from build123d import *

# Parameters (mm, degrees)
SKETCH1_R           = 12.5
BOSS_EXTRUDE1_DEPTH = 180
BOSS_EXTRUDE2_DEPTH = 20
SKETCH3_W           = 30.675059353
SKETCH3_H           = 4.752473984
CUT_EXTRUDE1_DEPTH  = 15


with BuildPart() as part:
    # Sketch1 → Boss-Extrude1 (new body)
    with BuildSketch(Plane.XY):
        with Locations(Location((0, 0, 0), (0, 0, 180))):
            Circle(SKETCH1_R)
    extrude(amount=BOSS_EXTRUDE1_DEPTH)

    # Sketch2 → Boss-Extrude2 (add)
    with BuildSketch(Plane.XY.offset(180)):
        Polygon((20.501198272, 0), (10.250599136, 17.754558511), (-10.250599136, 17.754558511), (-20.501198272, 0), (-10.250599136, -17.754558511), (10.250599136, -17.754558511), align=None)
    extrude(amount=BOSS_EXTRUDE2_DEPTH)

    # Sketch3 → Cut-Extrude1 (cut)
    with BuildSketch(Plane.XY.offset(200)):
        with Locations((0.504050272, -0.180017954)):
            Rectangle(SKETCH3_W, SKETCH3_H)
    extrude(amount=-CUT_EXTRUDE1_DEPTH, mode=Mode.SUBTRACT)


solid = part.part
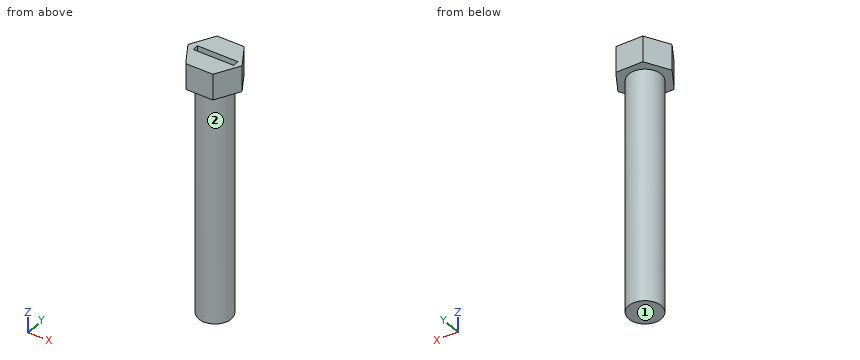
The listing builds one solid part. Answer for the finished solid, in the listing's coordinates (mm). Face numbers are marked on the shaded views. A direction names the side the tool comes from. Round coordinates to 2 decimals unless told otherwise and drop trailing zeros. Order: outer loops, then holes, each group sorted by start corner. A loop starts at its lowest first (then second) coordinate and runs counter-clockwise, first axis right, second up. Notation, with made-up numbers: M 13,22.25 L 61,22.25 A23 ccw 61,54.25 Z; hole C 47.25,57.5 d1. An arc over 180 degrees is marked long. Answer in a Markdown table with one row per item. Add a question column.
1) The part is cut by section A-A on x = 0. Determine the outline of the cut face in (y, z), plus the area to 3 significant figures.
2) Which of the six approach directions +Z, -Z, +X, -X, +Y, -Y give full straight-line access (tool end or side, diameter ignored) to the marked faces 1 and 2?
3) The part is cut by section B-B on z = 89. Determine the outline of the cut face in (x, y).
4) The part is cut by section C-C on y = 8. Determine the outline of the cut face in (x, z), plus the area to 3 significant figures.
5) Flat-ended cylindrical pins translate along their axes: pin 1 Ø12 at (x, z) = (6, 132.5) entering from -Y; pin 2 Ø1 at (y, z) = (-8, 100) entering from +X; pin 3 Ø1 at (x, y) = (10, -10) entering from -Z. Find the tip coordinate at first contact, or state that the pin passes through.
6) Consider line 1 along Z through (x, y) = (-12.5, -6.5); line 2 along Z through (x, y) = (3.5, -1); line 3 along X through (y, z) = (-1, 125). Determine where each line is inside the solid, lowest interval first. Write a range as from..to.
7) The part is cut by section D-D on y = -7.5. Determine the outline of the cut face in (x, z).
Findings below:
| question | item | result |
|---|---|---|
| 1 | outline | M -17.75,180 L -12.5,180 L -12.5,0 L 12.5,0 L 12.5,180 L 17.75,180 L 17.75,200 L 2.2,200 L 2.2,185 L -2.56,185 L -2.56,200 L -17.75,200 Z |
| 1 | area | 5,140 mm² |
| 2 | face 1 | -Z, +X, -X, +Y, -Y |
| 2 | face 2 | -Z |
| 3 | outline | C 0,0 d25 |
| 4 | outline | M -15.88,180 L -9.6,180 L -9.6,0 L 9.6,0 L 9.6,180 L 15.88,180 L 15.88,200 L -15.88,200 Z |
| 4 | area | 4,090 mm² |
| 5 | pin 1 | stops at y = -12.5 |
| 5 | pin 2 | stops at x = 10 |
| 5 | pin 3 | stops at z = 180 |
| 6 | line 1 | z = 180..200 |
| 6 | line 2 | z = 0..185 |
| 6 | line 3 | x = -12.46..12.46 |
| 7 | outline | M -16.17,180 L -10,180 L -10,0 L 10,0 L 10,180 L 16.17,180 L 16.17,200 L -16.17,200 Z |
